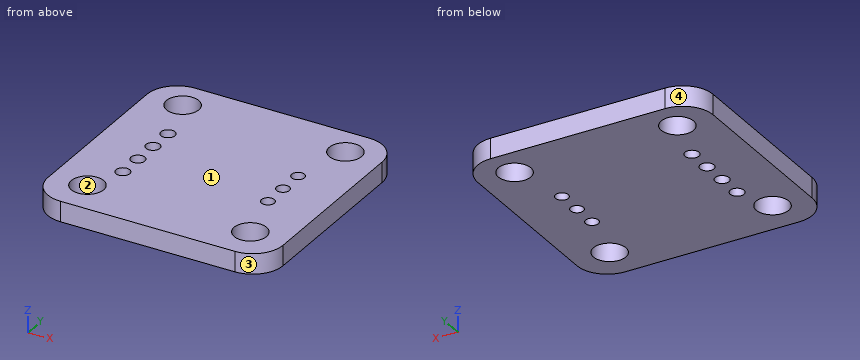
```python
from build123d import *

# Parameters (mm, degrees)
SKETCH1_W           = 23.2
SKETCH1_H           = 22.7
SKETCH1_R           = 1.6
BOSS_EXTRUDE1_DEPTH = 2
FILLET1_R           = 3
SKETCH2_R           = 0.633596253
SKETCH2_R_2         = 0.690319611
CUT_EXTRUDE1_DEPTH  = 17.526342483


with BuildPart() as part:
    # Sketch1 → Boss-Extrude1 (new body)
    with BuildSketch(Plane.XY):
        with Locations((-0.002931945, -0.247067135)):
            Rectangle(SKETCH1_W, SKETCH1_H)
        with Locations((-8.029814258, 8.024213837)):
            Circle(SKETCH1_R, mode=Mode.SUBTRACT)
        with Locations((8.021282811, 8.026881394)):
            Circle(SKETCH1_R, mode=Mode.SUBTRACT)
        with Locations((8.023950367, -8.024215675)):
            Circle(SKETCH1_R, mode=Mode.SUBTRACT)
        with Locations((-8.027146702, -8.026883232)):
            Circle(SKETCH1_R, mode=Mode.SUBTRACT)
    extrude(amount=BOSS_EXTRUDE1_DEPTH)

    # Fillet1
    fillet1_edges = [part.edges().sort_by_distance(p)[0] for p in [
        (11.597068055, -11.597067135, 1),
        (-11.602931945, -11.597067135, 1),
        (-11.602931945, 11.102932865, 1),
        (11.597068055, 11.102932865, 1),
    ]]
    fillet(fillet1_edges, radius=FILLET1_R)

    # Sketch2 → Cut-Extrude1 (cut, through all)
    with BuildSketch(Plane.XY.offset(2)):
        with Locations((6.647068055, -2.697067135)):
            Circle(SKETCH2_R)
        with Locations((6.647068055, -0.157067135)):
            Circle(SKETCH2_R)
        with Locations((6.647068055, 2.382932865)):
            Circle(SKETCH2_R)
        with Locations((-6.602931945, -4.497067135)):
            Circle(SKETCH2_R_2)
        with Locations((-6.602931945, -1.957067135)):
            Circle(SKETCH2_R_2)
        with Locations((-6.602931945, 0.582932865)):
            Circle(SKETCH2_R_2)
        with Locations((-6.602931945, 3.122932865)):
            Circle(SKETCH2_R_2)
    extrude(amount=-CUT_EXTRUDE1_DEPTH, mode=Mode.SUBTRACT)


solid = part.part
```
The model under review builds one solid part; all positions refer to its coordinate system, in mm. Face numbers are marked on the shaded views. Coordinates: 2 decimals unless noted, no trailing zeros. Order: outer loops, then holes, each group sorted by start corner. A loop starts at its lowest first (then second) coordinate and runs counter-clockwise, first axis right, second up. Notation, with made-up numbers: (40, -40) -> (84, -40) arc R18 cw to (84, -18) -> close; hole circle Ø7 at (69, -5.75). An arc over 180 degrees is marked (long way). Answer in a Markdown table with one row per item. Add a question column.
Item 1: We need section D-D on y = -3. Write out the cut boundary in (x, z).
Item 2: To check wall thickness, follow probe 1 along X at (y, z) = (-8, 1.05); probe 2 along Y at (x, z) = (-9.25, 0.7); probe 3 along Y at (x, z) = (7, 1.4). State the ranges of each line that lie inside material, in increasing order.
Item 3: We need section C-C on z = 0.5. Give the number of separate pieces and of enclosed holes in the cut face, plus the area to 3 significant figures.
Item 4: We need section B-B on x = 7. Write out the cut boundary in (y, z).
Item 5: We need section A-A on y = 8.5. Write out the cut boundary in (x, z), plus the area to 3 significant figures.
Item 6: Mouldability with a two-part tool opening along X and no side actions: class the marked faces 1, 2, 3 and 4 as +X half, -X half, draft (parallel to the pull), parting line (faces both ways), or undercut.
Item 7: Clearance check with flat-ended pins moving along their axes: pin 1 (1 mm diameter, centred on x = 6.65, y = 2.38, fed in from -Z); pin 2 (2 mm diameter, centred on x = -6.6, y = -4.5, fed in from -Z). State where each tip first meets the part, or that it passes through.
Final values:
| question | item | result |
|---|---|---|
| 1 | outline | (-11.6, 0) -> (6.09, 0) -> (6.09, 2) -> (-11.6, 2) -> close; (7.2, 0) -> (11.6, 0) -> (11.6, 2) -> (7.2, 2) -> close |
| 2 | probe 1 | x = -11.6 to -9.63, -6.43 to 6.42, 9.62 to 11.6 |
| 2 | probe 2 | y = -11.53 to -9.06, -7 to 6.99, 9.06 to 11.03 |
| 2 | probe 3 | y = -11.6 to -9.25, -6.79 to -3.22, -2.17 to -0.68, 0.37 to 1.86, 2.91 to 6.8, 9.26 to 11.1 |
| 3 | separate pieces | 1 |
| 3 | enclosed holes | 11 |
| 3 | area | 477 mm2 |
| 4 | outline | (-11.6, 0) -> (-9.25, 0) -> (-9.25, 2) -> (-11.6, 2) -> close; (-6.79, 0) -> (-3.22, 0) -> (-3.22, 2) -> (-6.79, 2) -> close; (-2.17, 0) -> (-0.68, 0) -> (-0.68, 2) -> (-2.17, 2) -> close; (0.37, 0) -> (1.86, 0) -> (1.86, 2) -> (0.37, 2) -> close; (2.91, 0) -> (6.8, 0) -> (6.8, 2) -> (2.91, 2) -> close; (9.26, 0) -> (11.1, 0) -> (11.1, 2) -> (9.26, 2) -> close |
| 5 | outline | (-11.58, 0) -> (-9.56, 0) -> (-9.56, 2) -> (-11.58, 2) -> close; (-6.5, 0) -> (6.49, 0) -> (6.49, 2) -> (-6.5, 2) -> close; (9.55, 0) -> (11.57, 0) -> (11.57, 2) -> (9.55, 2) -> close |
| 5 | area | 34.1 mm2 |
| 6 | face 1 | draft |
| 6 | face 2 | undercut |
| 6 | face 3 | +X half |
| 6 | face 4 | -X half |
| 7 | pin 1 | passes through |
| 7 | pin 2 | stops at z = 0 |
